from build123d import *

# Parameters (mm, degrees)
SKETCH_2_R          = 2.15
CUT_EXTRUDE_1_DEPTH = 10


with BuildPart() as part:
    # 草图1 → 旋转1 (revolve)
    with BuildSketch(Plane.XY, mode=Mode.PRIVATE) as revolve_1_sk:
        Polygon((75.5, 0), (88.9, 0), (88.9, 6.1), (75.5, 6.1), (75.5, 8.05), (72.5, 8.05), (72.5, -1.95), (75.5, -1.95), align=None)
    revolve(revolve_1_sk.sketch.rotate(Axis((0, 0, 0), (0, 1, 0)), 90), axis=Axis((0, 0, 0), (0, 1, 0)))

    # 草图2 → 切除-拉伸1 (cut)
    with BuildSketch(Plane(origin=(0, 6.1, 0), x_dir=(1, 0, 0), z_dir=(0, 1, 0))):
        with Locations(Location((-83.9, 0, 0), (0, 0, 270))):
            Circle(SKETCH_2_R)
        with Locations(Location((-59.326258942, 59.326258942, 0), (0, 0, 270))):
            Circle(SKETCH_2_R)
        with Locations(Location((0, 83.9, 0), (0, 0, 270))):
            Circle(SKETCH_2_R)
        with Locations(Location((59.326258942, 59.326258942, 0), (0, 0, 270))):
            Circle(SKETCH_2_R)
        with Locations(Location((83.9, 0, 0), (0, 0, 270))):
            Circle(SKETCH_2_R)
        with Locations(Location((59.326258942, -59.326258942, 0), (0, 0, 270))):
            Circle(SKETCH_2_R)
        with Locations(Location((0, -83.9, 0), (0, 0, 270))):
            Circle(SKETCH_2_R)
        with Locations(Location((-59.326258942, -59.326258942, 0), (0, 0, 270))):
            Circle(SKETCH_2_R)
    extrude(amount=-CUT_EXTRUDE_1_DEPTH, mode=Mode.SUBTRACT)


solid = part.part
Geometry: final body of the model. Coordinates: model frame, mm. A direction names the side the tool comes from. Round coordinates to 2 decimals unless told otherwise and drop trailing zeros. Loops run counter-clockwise (first coordinate to the right, second up) from the corner with the lowest first, then second, coordinate; pieces in that order, holes last. Notation, with made-up numbers: (-23.5, 87.25) -> (13.5, 87.25) arc R31 cw to (13.5, 113.25) -> close; hole circle Ø6 at (0.5, -36). An arc over 180 degrees is marked (long way). One line per question, with ' | ' between items. Start each with the question number.
1. Line query: line 1 along X through (y, z) = (6.5, 1); line 2 along Z through (x, y) = (-58, 4.25); line 3 along X through (y, z) = (-1.25, -52). Output: solid intervals per line, ascending. Write a range as [from, to].
2. Set-up query: faces 1 (the face through (-22.678, 7.089, -72.014)), 2 (the face through (-67.5, 8.05, 28.3)), 3 (the face through (-20, 0, -73)). Return all of +Z, -Z, +X, -X, +Y, -Y with unobstructed straight access to the full face (end or side cutting, diameter ignored); none if empty.
3. Section C-C on x = 83.9. Output: boundary loops of the cut face in (y, z).
4. Section B-B on x = 0. Output: boundary loops of the cut face in (y, z), and give its area (3 significant figures).
5. Section D-D on z = -83.9. Output: boundary loops of the cut face in (x, y).
6. Contact query for flat-ended pins moving along their axis: pin 1 (5 mm diameter, centred on y = 2, z = 51.5, fed in from -X); pin 2 (5 mm diameter, centred on x = -59.33, z = 59.33, fed in from -Y); pin 3 (2.5 mm diameter, centred on x = 0, z = -83.9, fed in from +Y); pin 4 (1 mm diameter, centred on y = 2.5, z = -63.5, fed in from +X). Output: stop coordinate, or through.
7. Mould query, pull axis X, two halves, no side actions, for faces 4 (the face through (81.99, 3.09, 0.99)), 5 (the face through (-22.678, -0.961, -72.014)), 6 (the face through (-20, 6.1, 73)). Classes: pulls with the +X half, pulls with the -X half, needs draft (parallel to the pull), parting line crosses it, or undercut.
8. Section A-A on z = 0. Output: boundary loops of the cut face in (x, y), and give its area (3 significant figures).
Returned:
1) line 1: x = [-75.49, -72.49], [72.49, 75.49] | line 2: z = [-67.37, -61.02], [-57.63, -43.5], [43.5, 57.63], [61.02, 67.37] | line 3: x = [-54.74, -50.52], [50.52, 54.74]
2) face 1: +Y | face 2: +Z, -Z, +X, -X, +Y | face 3: -Y
3) outline: (0, -29.39) -> (6.1, -29.39) -> (6.1, -2.15) -> (0, -2.15) -> close; (0, 2.15) -> (6.1, 2.15) -> (6.1, 29.39) -> (0, 29.39) -> close
4) outline: (-1.95, -75.5) -> (0, -75.5) -> (0, -81.75) -> (6.1, -81.75) -> (6.1, -75.5) -> (8.05, -75.5) -> (8.05, -72.5) -> (-1.95, -72.5) -> close; (-1.95, 72.5) -> (8.05, 72.5) -> (8.05, 75.5) -> (6.1, 75.5) -> (6.1, 81.75) -> (0, 81.75) -> (0, 75.5) -> (-1.95, 75.5) -> close; (0, -88.9) -> (6.1, -88.9) -> (6.1, -86.05) -> (0, -86.05) -> close; (0, 86.05) -> (6.1, 86.05) -> (6.1, 88.9) -> (0, 88.9) -> close | area: 171 mm2
5) outline: (-29.39, 0) -> (-2.15, 0) -> (-2.15, 6.1) -> (-29.39, 6.1) -> close; (2.15, 0) -> (29.39, 0) -> (29.39, 6.1) -> (2.15, 6.1) -> close
6) pin 1: stops at x = -74.18 | pin 2: stops at y = 0 | pin 3: passes through | pin 4: stops at x = 62.72
7) face 4: undercut | face 5: parting line crosses it | face 6: needs draft
8) outline: (-88.9, 0) -> (-86.05, 0) -> (-86.05, 6.1) -> (-88.9, 6.1) -> close; (-81.75, 0) -> (-75.5, 0) -> (-75.5, -1.95) -> (-72.5, -1.95) -> (-72.5, 8.05) -> (-75.5, 8.05) -> (-75.5, 6.1) -> (-81.75, 6.1) -> close; (72.5, -1.95) -> (75.5, -1.95) -> (75.5, 0) -> (81.75, 0) -> (81.75, 6.1) -> (75.5, 6.1) -> (75.5, 8.05) -> (72.5, 8.05) -> close; (86.05, 0) -> (88.9, 0) -> (88.9, 6.1) -> (86.05, 6.1) -> close | area: 171 mm2
